Input: dimensioned drawing with shaded views. Units: mm. Origin: part minimum x, y, z. Coordinates: 2 decimals unless noted, no trailing zeros. Loops run counter-clockwise (first coordinate to the right, second up) from the corner with the lowest first, then second, coordinate; pieces in that order, holes last. Notation, with made-up numbers: (75.25, 56.5) - (93.25, 56.5) arc R26 cw to (93.25, 92.5) - close; hole circle Ø3 at (-7, 47.25). An arc over 180 degrees is marked (long way). Write item = value, one per line. Start each with the question number.
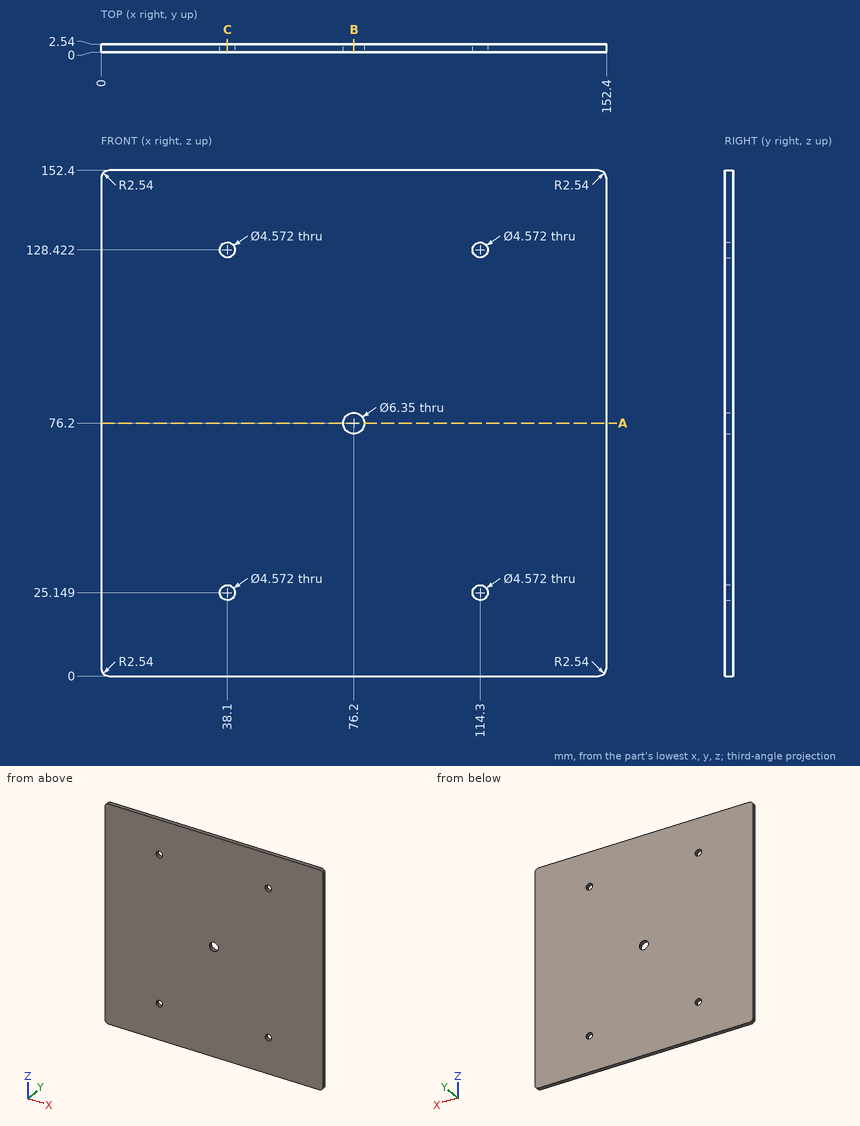
Item 1: Ray query, line 1 (Z direction, x = 38.1, y = 1.3) (1 decimal); line 2 (Z direction, x = 76.2, y = 1.85) (1 decimal); line 3 (X direction, y = 0.2, z = 26). Return the intervals inside material, ascending.
Item 2: Cut plane C-C on x = 38.1. Return loops of the section in (y, z) (1 decimal).
Item 3: Pin query (flat end, axial travel): pin 1 (10 mm diameter, centred on x = 76.2, z = 76.2, fed in from +Y); pin 2 (3.5 mm diameter, centred on x = 38.1, z = 128.42, fed in from -Y). Return the tip coordinate at first contact, or that it passes through.
Item 4: Cut plane A-A on z = 76.2. Return loops of the section in (x, y) (1 decimal), plus the area to 3 significant figures.
Item 5: Cut plane B-B on x = 76.2. Return loops of the section in (y, z) (1 decimal).
Recorded:
q1.line_1 = 0 to 22.9, 27.4 to 126.1, 130.7 to 152.4
q1.line_2 = 0 to 73, 79.4 to 152.4
q1.line_3 = 0 to 35.98, 40.22 to 112.18, 116.42 to 152.4
q2.outline = (0, 0) - (2.5, 0) - (2.5, 22.9) - (0, 22.9) - close; (0, 27.4) - (2.5, 27.4) - (2.5, 126.1) - (0, 126.1) - close; (0, 130.7) - (2.5, 130.7) - (2.5, 152.4) - (0, 152.4) - close
q3.pin_1 = 2.54
q3.pin_2 = through
q4.outline = (0, 0) - (73, 0) - (73, 2.5) - (0, 2.5) - close; (79.4, 0) - (152.4, 0) - (152.4, 2.5) - (79.4, 2.5) - close
q4.area = 371 mm²
q5.outline = (0, 0) - (2.5, 0) - (2.5, 73) - (0, 73) - close; (0, 79.4) - (2.5, 79.4) - (2.5, 152.4) - (0, 152.4) - close
